from build123d import *

# Parameters (mm, degrees)
F1_DEPTH = 35


with BuildPart() as f1:
    # F0 (on Front) → F1 (new body)
    with BuildSketch(Plane.XZ):
        Polygon((-6.12, 3.2), (-6.12, 0), (-4.1, 0), (-4.1, -5), (4.1, -5), (4.1, 0), (6.12, 0), (6.12, 3.2), (0, 3.2), align=None)
        Polygon((4.1, -5), (-4.1, -5), (-11.1, -5), (-15, -5), (-15, -40), (15, -40), (15, -5), (11.1, -5), align=None)
    extrude(amount=F1_DEPTH)


solid = f1.part
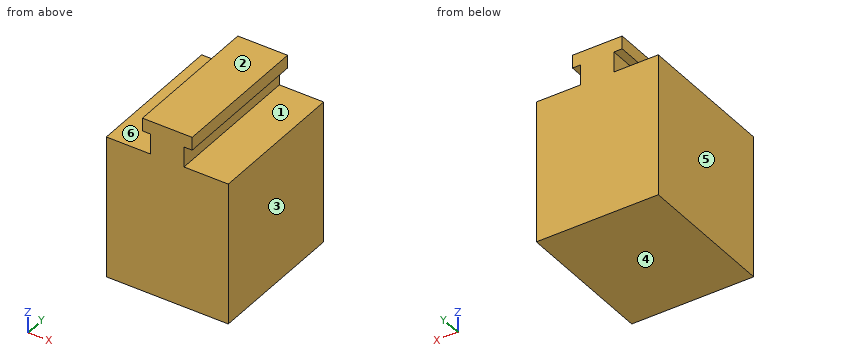
Check sheet for the modelled part. Datum: model origin and axes. Units: mm. Face numbers are marked on the shaded views. A direction names the side the tool comes from. Give positions to 0.01 mm unless a question says otherwise; leave off trailing zeros. Write each loop counter-clockwise with the first axis right and the second up, starting at its lowest first coordinate (ties: lowest second). Pieces come first, ordered by that corner, then holes. Notation, with made-up numbers: (3, 46) -> (8, 46) arc R20 cw to (8, 82) -> close; hole circle Ø5 at (65.5, 2). An arc over 180 degrees is marked (long way). One line per item, written item: value. Start each with the question number.
Item 1: Section check C-C on z = -2. Record the cut outline in (x, y), then the cut area to 3 significant figures.
Item 2: Material ranges on probe 1 along Z at (x, y) = (-5, -14.5); probe 2 along Z at (x, y) = (-10.5, -18); probe 3 along X at (y, z) = (-11, -4), recorded low to high. Write a range as from..to.
Item 3: Section check B-B on x = -7. Record the cut outline in (y, z).
Item 4: Draft check along Z on the marked faces 1, 2, 3 and 4. Enter one of: +Z half, -Z half, draft (parallel to the pull), parting line (faces both ways), or undercut.
Item 5: Gauge pin test, flat ends, axial feed: pin 1 (4 mm diameter, centred on x = -11.5, y = -21.5, fed in from +Z); pin 2 (1.5 mm diameter, centred on y = -23, z = -1.5, fed in from -X); pin 3 (1 mm diameter, centred on y = -11, z = 1, fed in from +X). Record the tip position at first contact, or that the pin passes through.
Item 6: Tool access check on the marked faces 5 and 6. Record the directions out of +Z, -Z, +X, -X, +Y, -Y that give a thin tool (end or side, any length) a straight path to the whole face; none if there is none.
Item 7: Section check A-A on y = -8.5. Record the cut outline in (x, z), then the cut area to 3 significant figures.
Results list:
1. outline: (-4.1, -35) -> (4.1, -35) -> (4.1, 0) -> (-4.1, 0) -> close
1. area: 287 mm²
2. probe 1: -40..-5, 0..3.2
2. probe 2: -40..-5
2. probe 3: -4.1..4.1
3. outline: (-35, -40) -> (0, -40) -> (0, -5) -> (-35, -5) -> close
4. face 1: undercut
4. face 2: +Z half
4. face 3: draft
4. face 4: -Z half
5. pin 1: z = -5
5. pin 2: x = -4.1
5. pin 3: x = 6.12
6. face 5: +Z, -Z, -X, +Y, -Y
6. face 6: -X, +Y, -Y
7. outline: (-15, -40) -> (15, -40) -> (15, -5) -> (4.1, -5) -> (4.1, 0) -> (6.12, 0) -> (6.12, 3.2) -> (-6.12, 3.2) -> (-6.12, 0) -> (-4.1, 0) -> (-4.1, -5) -> (-15, -5) -> close
7. area: 1,130 mm²
